Input: dimensioned drawing with shaded views. Units: mm. Origin: part minimum x, y, z. A direction names the side the tool comes from. Give positions to 0.01 mm unless a question says otherwise; leave off trailing zeros. Loops run counter-clockwise (first coordinate to the right, second up) from the corner with the lowest first, then second, coordinate; pieces in that order, holes last. Notation, with made-up numbers: M 26.25,89 L 60.25,89 A15 ccw 60.25,117 Z; hole C 39.25,-18 d6. An arc over 180 degrees is marked long. Answer in a Markdown table with one row per item.
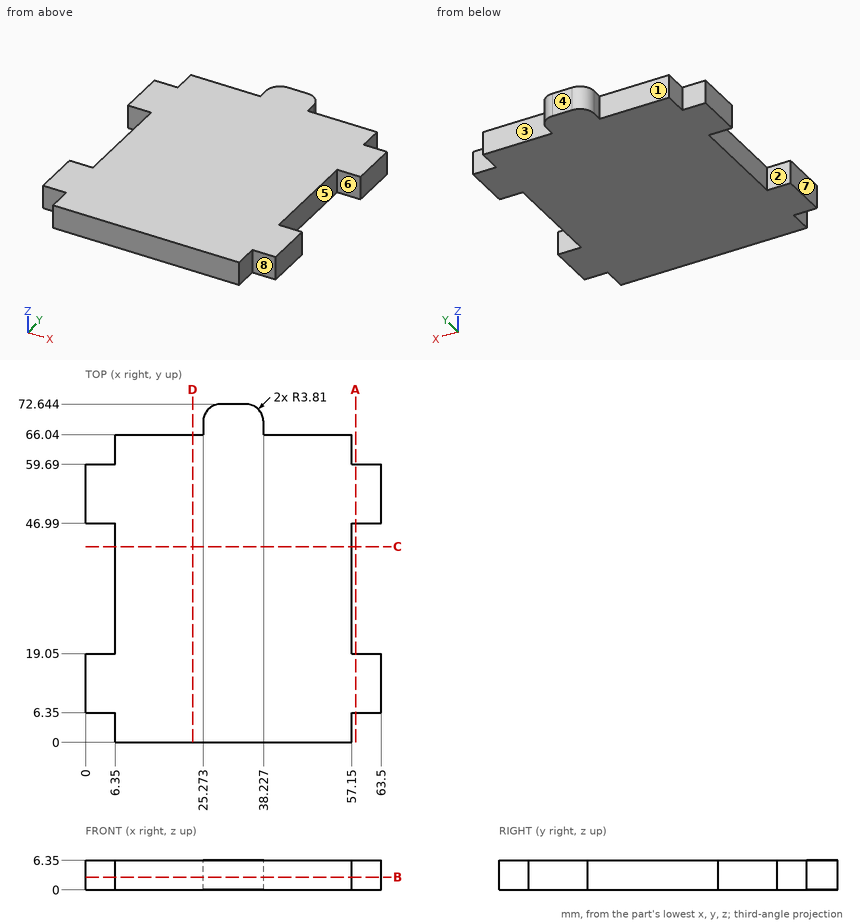
Q1. Section query B-B (z = 2.75). Output: boundary loops of the cut face in (x, y).
Values follow:
| item | result |
|---|---|
| outline | M 0,6.35 L 6.35,6.35 L 6.35,0 L 57.15,0 L 57.15,6.35 L 63.5,6.35 L 63.5,19.05 L 57.15,19.05 L 57.15,46.99 L 63.5,46.99 L 63.5,59.69 L 57.15,59.69 L 57.15,66.04 L 38.23,66.04 L 38.23,68.83 A3.81 ccw 34.42,72.64 L 29.08,72.64 A3.81 ccw 25.27,68.83 L 25.27,66.04 L 6.35,66.04 L 6.35,59.69 L 0,59.69 L 0,46.99 L 6.35,46.99 L 6.35,19.05 L 0,19.05 Z |
Q2. Mould query, pull axis Y, two halves, no side actions, for the marked faces 6, 7 and 8. Classes: +Y half, -Y half, draft (parallel to the pull), parting line (faces both ways), or undercut.
Values follow:
| item | result |
|---|---|
| face 6 | undercut |
| face 7 | draft |
| face 8 | -Y half |
Q3. Section query D-D (x = 23). Output: boundary loops of the cut face in (y, z), plus the area to 3 significant figures.
Values follow:
| item | result |
|---|---|
| outline | M 0,0 L 66.04,0 L 66.04,6.35 L 0,6.35 Z |
| area | 419 mm^2 |
Q4. Contact query for flat-ended pins moving along their axis: pin 1 Ø1.4 at (y, z) = (68, 2.5) entering from +X; pin 2 Ø1.9 at (y, z) = (3.5, 3.5) entering from -X; pin 3 Ø1.9 at (x, z) = (3, 3) entering from +Y. Output: stop coordinate, or through.
Values follow:
| item | result |
|---|---|
| pin 1 | x = 38.23 |
| pin 2 | x = 6.35 |
| pin 3 | y = 59.69 |
Q5. Section query A-A (x = 58). Output: boundary loops of the cut face in (y, z), plus the area to 3 significant figures.
Values follow:
| item | result |
|---|---|
| outline | M 6.35,0 L 19.05,0 L 19.05,6.35 L 6.35,6.35 Z; M 46.99,0 L 59.69,0 L 59.69,6.35 L 46.99,6.35 Z |
| area | 161 mm^2 |
Q6. Section query C-C (y = 42). Output: boundary loops of the cut face in (x, z).
Values follow:
| item | result |
|---|---|
| outline | M 6.35,0 L 57.15,0 L 57.15,6.35 L 6.35,6.35 Z |
Q7. Ray query, probe 1 along Y at (x, z) = (4.5, 6); probe 2 along X at (y, z) = (35, 2.75); probe 3 along Y at (x, z) = (53.5, 0.5). Return the intervals inside material, ascending. Write a range as from..to.
Values follow:
| item | result |
|---|---|
| probe 1 | 6.35..19.05, 46.99..59.69 |
| probe 2 | 6.35..57.15 |
| probe 3 | 0..66.04 |
Q8. Reachability of the marked faces 1, 2, 3, 4 and 5 from +Z, -Z, +X, -X, +Y, -Y: full face, straight path, thin tool, end or side. Return the list, or none.
Values follow:
| item | result |
|---|---|
| face 1 | +Z, -Z, -X, +Y |
| face 2 | +Z, -Z, -X |
| face 3 | +Z, -Z, +X, +Y |
| face 4 | +Z, -Z, +X, -X, +Y |
| face 5 | +Z, -Z, +X |
